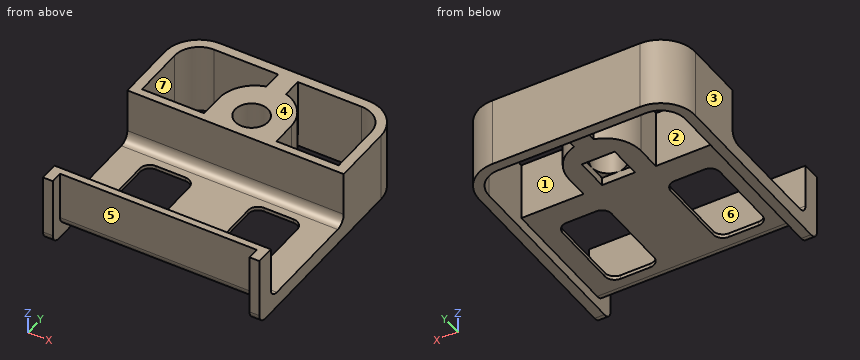
from build123d import *

# Parameters (mm, degrees)
F1_DEPTH = 18.034
F3_W     = 8.509
F3_H     = 8.509
F4_DEPTH = 2.032
F5_R     = 4.2545
F6_DEPTH = 12.954
F8_DEPTH = 55.881
F9_R     = 2.54


with BuildPart() as f1:
    # F0 (on Top) → F1 (new body)
    with BuildSketch(Plane.XY):
        with BuildLine():
            Line((-27.94, 21.209), (-27.94, -30.099))
            Line((-27.94, -30.099), (-25.4, -30.099))
            Line((-25.4, -30.099), (-25.4, 21.209))
            ThreePointArc((-25.4, 21.209), (-23.540128, 25.699128), (-19.05, 27.559))
            Line((-19.05, 27.559), (19.05, 27.559))
            ThreePointArc((19.05, 27.559), (23.540128, 25.699128), (25.4, 21.209))
            Line((25.4, 21.209), (25.4, -30.099))
            Line((25.4, -30.099), (27.94, -30.099))
            Line((27.94, -30.099), (27.94, 21.209))
            ThreePointArc((27.94, 21.209), (25.336179, 27.495179), (19.05, 30.099))
            Line((19.05, 30.099), (-19.05, 30.099))
            ThreePointArc((-19.05, 30.099), (-25.336179, 27.495179), (-27.94, 21.209))
        make_face()
    extrude(amount=F1_DEPTH)

    # F3 (on offset) → F4 (join)
    with BuildSketch(Plane.XY.offset(3.048)):
        with BuildLine():
            Line((-25.4, 7.493), (-25.4, -27.051))
            Line((-25.4, -27.051), (25.4, -27.051))
            Line((25.4, -27.051), (25.4, 7.493))
            Line((25.4, 7.493), (9.3345, 7.493))
            Line((9.3345, 7.493), (9.3345, 13.828916))
            ThreePointArc((9.3345, 13.828916), (7.382472, 19.335437), (2.54, 22.60387))
            Line((2.54, 22.60387), (2.54, 27.559))
            Line((2.54, 27.559), (-2.54, 27.559))
            Line((-2.54, 27.559), (-2.54, 22.60387))
            ThreePointArc((-2.54, 22.60387), (-7.382472, 19.335437), (-9.3345, 13.828916))
            Line((-9.3345, 13.828916), (-9.3345, 7.493))
            Line((-9.3345, 7.493), (-25.4, 7.493))
        make_face()
        with BuildLine():
            ThreePointArc((-20.32, -1.651), (-19.576051, 0.145051), (-17.78, 0.889))
            Line((-17.78, 0.889), (-10.16, 0.889))
            ThreePointArc((-10.16, 0.889), (-8.363949, 0.145051), (-7.62, -1.651))
            Line((-7.62, -1.651), (-7.62, -19.431))
            ThreePointArc((-7.62, -19.431), (-8.363949, -21.227051), (-10.16, -21.971))
            Line((-10.16, -21.971), (-17.78, -21.971))
            ThreePointArc((-17.78, -21.971), (-19.576051, -21.227051), (-20.32, -19.431))
            Line((-20.32, -19.431), (-20.32, -1.651))
        make_face(mode=Mode.SUBTRACT)
        with BuildLine():
            ThreePointArc((7.62, -1.651), (8.363949, 0.145051), (10.16, 0.889))
            Line((10.16, 0.889), (17.78, 0.889))
            ThreePointArc((17.78, 0.889), (19.576051, 0.145051), (20.32, -1.651))
            Line((20.32, -1.651), (20.32, -19.431))
            ThreePointArc((20.32, -19.431), (19.576051, -21.227051), (17.78, -21.971))
            Line((17.78, -21.971), (10.16, -21.971))
            ThreePointArc((10.16, -21.971), (8.363949, -21.227051), (7.62, -19.431))
            Line((7.62, -19.431), (7.62, -1.651))
        make_face(mode=Mode.SUBTRACT)
        with Locations((0, 12.2555)):
            Rectangle(F3_W, F3_H, mode=Mode.SUBTRACT)
    extrude(amount=F4_DEPTH)

    # F5 (on face) → F6 (join, through all)
    with BuildSketch(Plane.XY.offset(5.08)):
        with BuildLine():
            Line((-9.3345, 13.828916), (-9.3345, 7.493))
            Line((-9.3345, 7.493), (-25.4, 7.493))
            Line((-25.4, 7.493), (-25.4, -27.051))
            Line((-25.4, -27.051), (25.4, -27.051))
            Line((25.4, -27.051), (25.4, 7.493))
            Line((25.4, 7.493), (9.3345, 7.493))
            Line((9.3345, 7.493), (9.3345, 13.828916))
            ThreePointArc((9.3345, 13.828916), (7.382472, 19.335437), (2.54, 22.60387))
            Line((2.54, 22.60387), (2.54, 27.559))
            Line((2.54, 27.559), (-2.54, 27.559))
            Line((-2.54, 27.559), (-2.54, 22.60387))
            ThreePointArc((-2.54, 22.60387), (-7.382472, 19.335437), (-9.3345, 13.828916))
        make_face()
        with Locations((0, 12.2555)):
            Circle(F5_R, mode=Mode.SUBTRACT)
    extrude(amount=F6_DEPTH)

    # F7 (on face) → F8 (cut, through all)
    with BuildSketch(Plane.YZ.offset(27.94)):
        with BuildLine():
            Line((5.461, 18.034), (-25.273, 18.034))
            Line((-25.273, 18.034), (-25.273, 6.604))
            ThreePointArc((-25.273, 6.604), (-24.529051, 4.807949), (-22.733, 4.064))
            Line((-22.733, 4.064), (2.921, 4.064))
            ThreePointArc((2.921, 4.064), (4.717051, 4.807949), (5.461, 6.604))
            Line((5.461, 6.604), (5.461, 18.034))
        make_face()
    extrude(amount=-F8_DEPTH, mode=Mode.SUBTRACT)

    # F9
    f9_edges = [f1.edges().sort_by_distance(p)[0] for p in [
        (-26.67, -30.099, 0),
        (26.67, -30.099, 0),
        (0, -27.051, 3.048),
    ]]
    fillet(f9_edges, radius=F9_R)


solid = f1.part
Build history of the part. All positions in model axes, mm. Face numbers are marked on the shaded views. A direction names the side the tool comes from. Give positions to 0.01 mm unless a question says otherwise; leave off trailing zeros. Order: outer loops, then holes, each group sorted by start corner. A loop starts at its lowest first (then second) coordinate and runs counter-clockwise, first axis right, second up. Notation, with made-up numbers: M 14,62.5 L 53,62.5 A26 ccw 53,83.5 Z; hole C -1.5,-21 d8. An arc over 180 degrees is marked long. Use one line per item in the form item = value.
Q1. Pin check, flat tips, straight feed: P1, Ø10, axis at x = 16.5, y = -16.5, coming from the +Z side; P2, Ø10, axis at x = 19.5, y = -5.5, coming from the -Z side; P3, Ø3.5, axis at x = 1, y = 10.5, coming from the -Z side; P4, Ø1.1, axis at x = 14.5, z = 3.5, coming from the -Y side. Stop position of each tip, or through.
Conclusion:
P1 = 4.06
P2 = 3.05
P3 = through
P4 = -26.53
Q2. Slice it at C-C, the plane x = 11. Write the cut outline in (y, z), and give its area (3 significant figures).
Conclusion:
outline = M -27.05,5.59 A2.54 ccw -24.51,3.05 L -21.97,3.05 L -21.97,4.06 L -22.73,4.06 A2.54 cw -25.27,6.6 L -25.27,18.03 L -27.05,18.03 Z; M 0.89,3.05 L 7.49,3.05 L 7.49,18.03 L 5.46,18.03 L 5.46,6.6 A2.54 cw 2.92,4.06 L 0.89,4.06 Z; M 27.56,0 L 30.1,0 L 30.1,18.03 L 27.56,18.03 Z
area = 112 mm2
Q3. Slice it at B-B, the plane y = -11. Write the cut outline in (x, z).
Conclusion:
outline = M -27.94,0 L -25.4,0 L -25.4,3.05 L -20.32,3.05 L -20.32,4.06 L -27.94,4.06 Z; M -7.62,3.05 L 7.62,3.05 L 7.62,4.06 L -7.62,4.06 Z; M 20.32,3.05 L 25.4,3.05 L 25.4,0 L 27.94,0 L 27.94,4.06 L 20.32,4.06 Z
Q4. Which spindle directions (+Z, -Z, +X, -X, +Y, -Y) get a long thin tool onto all of the face, cutting with end or side? Do the marked faces 5, 6 and 7. Say none if no direction does.
Conclusion:
face_5 = +Z, -Z, -Y
face_6 = +Z, +X, -X
face_7 = -Z
Q5. Slice it at A-A, the plane z = 9.5. State how many separate pieces and enclosed holes the cut face has, and give its area (3 significant figures).
Conclusion:
separate_pieces = 2
enclosed_holes = 3
area = 674 mm2
Q6. Pull direction X, two halves, no side cores. Call the marked faces 1, 2, 3 and 4: released by +X, released by -X, zero draft, split by the parting line, or undercut.
Conclusion:
face_1 = undercut
face_2 = undercut
face_3 = released by -X
face_4 = zero draft
Q7. Slice it at D-D, the plane x = 1. Write the cut outline in (y, z), and give its area (3 significant figures).
Conclusion:
outline = M -27.05,5.59 A2.54 ccw -24.51,3.05 L 8,3.05 L 8,5.08 L 8.12,5.08 L 8.12,18.03 L 5.46,18.03 L 5.46,6.6 A2.54 cw 2.92,4.06 L -22.73,4.06 A2.54 cw -25.27,6.6 L -25.27,18.03 L -27.05,18.03 Z; M 16.39,5.08 L 16.51,5.08 L 16.51,3.05 L 27.56,3.05 L 27.56,0 L 30.1,0 L 30.1,18.03 L 16.39,18.03 Z
area = 312 mm2
Q8. Wall check: probe 1 along Y at (x, z) = (0, 11); probe 2 along Y at (x, z) = (10.5, 13.25); probe 3 along X at (y, z) = (21, 16.75). Give the ranges that are in metal, low to high.
Conclusion:
probe_1 = -27.05 to -25.27, 5.46 to 8, 16.51 to 30.1
probe_2 = -27.05 to -25.27, 5.46 to 7.49, 27.56 to 30.1
probe_3 = -27.94 to -25.4, -5.72 to 5.72, 25.4 to 27.94
